Verification items for the finished model (mm, model axes). Round coordinates to 2 decimals unless told otherwise and drop trailing zeros. Write each loop counter-clockwise with the first axis right and the second up, starting at its lowest first coordinate (ties: lowest second). Pieces come first, ordered by that corner, then holes. Notation, with made-up numbers: (41.5, 68.25) - (60.5, 68.25) arc R33 cw to (60.5, 98.25) - close; hole circle Ø2 at (-30, 56.5). An arc over 180 degrees is marked (long way). Answer as a JSON object with one key per item and string values.
```python
from build123d import *

# Parameters (mm, degrees)
SKIZZE1_W                       = 148
SKIZZE1_H                       = 158
AUFSATZ_LINEAR_AUSTRAGEN1_DEPTH = 5
SKIZZE2_W                       = 158
SKIZZE2_H                       = 50
AUFSATZ_LINEAR_AUSTRAGEN2_DEPTH = 5
SKIZZE3_W                       = 50
SKIZZE3_H                       = 168
AUFSATZ_LINEAR_AUSTRAGEN3_DEPTH = 5
SKIZZE4_R                       = 50
SCHNITT_LINEAR_AUSTRAGEN1_DEPTH = 5
SKIZZE5_W                       = 128
SKIZZE5_H                       = 138
SCHNITT_LINEAR_AUSTRAGEN2_DEPTH = 116.420968632
VERRUNDUNG1_R                   = 10


with BuildPart() as part:
    # Skizze1 → Aufsatz-Linear austragen1 (new body)
    with BuildSketch(Plane(origin=(0, 0, 0), x_dir=(1, 0, 0), z_dir=(0, 1, 0))):
        Rectangle(SKIZZE1_W, SKIZZE1_H)
    extrude(amount=AUFSATZ_LINEAR_AUSTRAGEN1_DEPTH)

    # Skizze2 → Aufsatz-Linear austragen2 (add)
    with BuildSketch(Plane(origin=(0, 5, 0), x_dir=(1, 0, 0), z_dir=(0, 1, 0))):
        Rectangle(SKIZZE2_W, SKIZZE2_H)
    extrude(amount=-AUFSATZ_LINEAR_AUSTRAGEN2_DEPTH)

    # Skizze3 → Aufsatz-Linear austragen3 (add)
    with BuildSketch(Plane(origin=(0, 5, 0), x_dir=(1, 0, 0), z_dir=(0, 1, 0))):
        Rectangle(SKIZZE3_W, SKIZZE3_H)
    extrude(amount=-AUFSATZ_LINEAR_AUSTRAGEN3_DEPTH)

    # Skizze4 → Schnitt-Linear austragen1 (cut)
    with BuildSketch(Plane(origin=(0, 5, 0), x_dir=(1, 0, 0), z_dir=(0, 1, 0))):
        with Locations(Location((0, 0, 0), (0, 0, 270))):
            Circle(SKIZZE4_R)
    extrude(amount=-SCHNITT_LINEAR_AUSTRAGEN1_DEPTH, mode=Mode.SUBTRACT)

    # Skizze5 → Schnitt-Linear austragen2 (cut, through all)
    with BuildSketch(Plane(origin=(0, 5, 0), x_dir=(1, 0, 0), z_dir=(0, 1, 0))):
        Rectangle(SKIZZE5_W, SKIZZE5_H)
    extrude(amount=-SCHNITT_LINEAR_AUSTRAGEN2_DEPTH, mode=Mode.SUBTRACT)

    # Verrundung1
    verrundung1_edges = [part.edges().sort_by_distance(p)[0] for p in [
        (64, 2.5, 69),
        (-64, 2.5, 69),
        (-64, 2.5, -69),
        (64, 2.5, -69),
    ]]
    fillet(verrundung1_edges, radius=VERRUNDUNG1_R)


solid = part.part
```
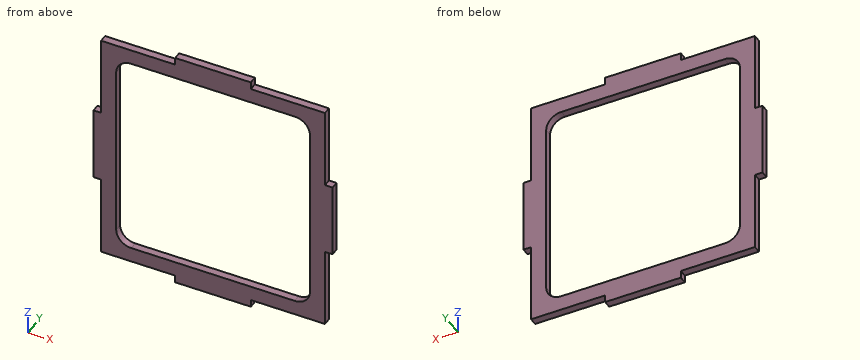
Q1. Material ranges on line 1 along X through (y, z) = (2.6, -30); line 2 along X through (y, z) = (3.2, -0.5); line 3 along Z through (x, y) = (-34, 4.7), recorded low to high. Write a range as [from, to].
Geometry check:
{"line 1": "x = [-74, -64], [64, 74]", "line 2": "x = [-79, -64], [64, 79]", "line 3": "z = [-79, -69], [69, 79]"}
Q2. Section check C-C, the plane y = 3.7. Record the cut outline in (x, z), then the cut area to 3 significant figures.
Geometry check:
{"outline": "(-79, -25) - (-74, -25) - (-74, -79) - (-25, -79) - (-25, -84) - (25, -84) - (25, -79) - (74, -79) - (74, -25) - (79, -25) - (79, 25) - (74, 25) - (74, 79) - (25, 79) - (25, 84) - (-25, 84) - (-25, 79) - (-74, 79) - (-74, 25) - (-79, 25) - close; hole (-64, -59) arc R10 ccw to (-54, -69) - (54, -69) arc R10 ccw to (64, -59) - (64, 59) arc R10 ccw to (54, 69) - (-54, 69) arc R10 ccw to (-64, 59) - close", "area": "6,810 mm2"}
Q3. Section check A-A, the plane x = -28. Record the cut outline in (y, z).
Geometry check:
{"outline": "(0, -79) - (5, -79) - (5, -69) - (0, -69) - close; (0, 69) - (5, 69) - (5, 79) - (0, 79) - close"}
Q4. Gauge pin test, flat ends, axial feed: P1, Ø1.5, axis at x = -75.5, y = 2.5, coming from the -Z side; P2, Ø2.5, axis at x = -76.5, y = 3, coming from the +Z side; P3, Ø2.5, axis at y = 2, z = 82, coming from the +X side. Record the tip position at first contact, or that the pin passes through.
Geometry check:
{"P1": "stops at z = -25", "P2": "stops at z = 25", "P3": "stops at x = 25"}
Q5. Section check B-B, the plane z = -1.5. Record the cut outline in (x, y), then the cut area to 3 significant figures.
Geometry check:
{"outline": "(-79, 0) - (-64, 0) - (-64, 5) - (-79, 5) - close; (64, 0) - (79, 0) - (79, 5) - (64, 5) - close", "area": "150 mm2"}
